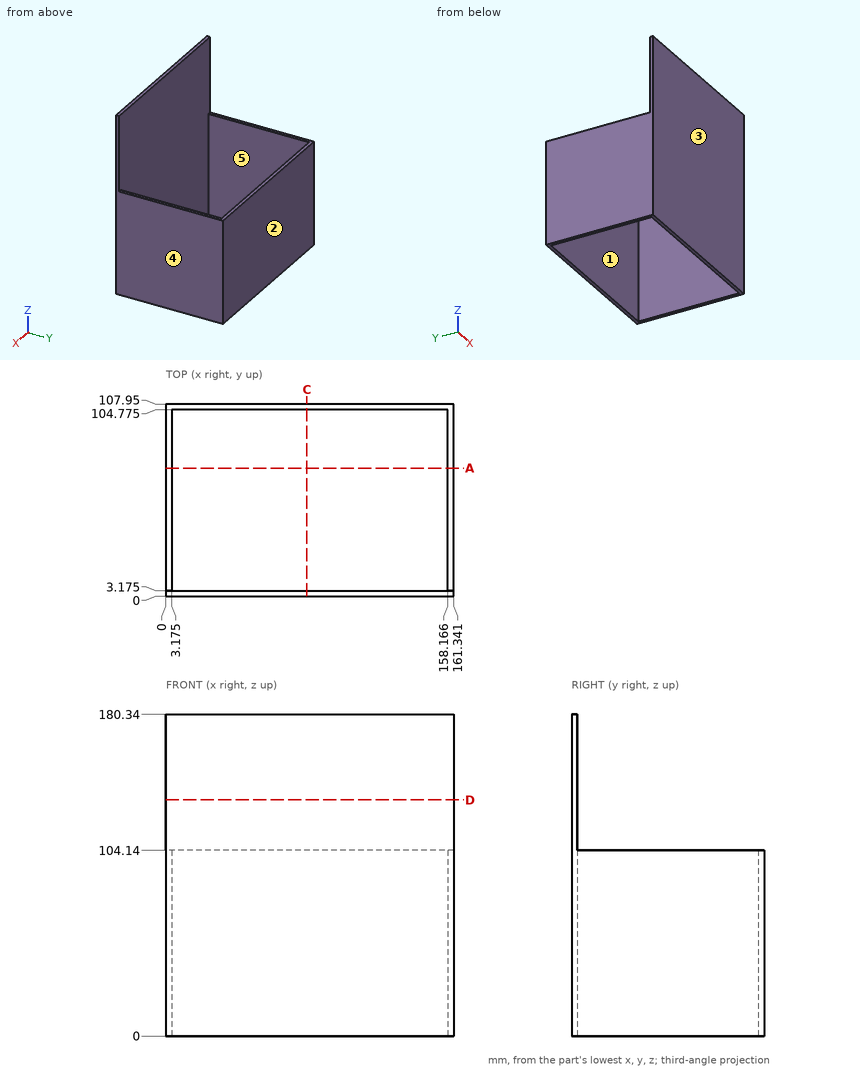
Geometry check sheet. Reference: drawing and pictorial views, mm from the part's lowest x, y, z. A direction names the side the tool comes from. Round coordinates to 2 decimals unless told otherwise and drop trailing zeros. Loops run counter-clockwise (first coordinate to the right, second up) from the corner with the lowest first, then second, coordinate; pieces in that order, holes last. Notation, with made-up numbers: (61, -17.5) - (117, -17.5) arc R19 cw to (117, 19.5) - close; hole circle Ø2 at (33.5, -24). An arc over 180 degrees is marked (long way). Use a Markdown table: item, result. Add a question column.
1. Release check for a two-part mould opening along X. For the marked faces 3, 4 and 5 record: released by +X, released by -X, zero draft, split by the parting line, or undercut.
2. Section check A-A, the plane y = 72. Record the boundary of the cut face in (x, z) (1 decimal), plus the area to 3 significant figures.
3. Gauge pin test, flat ends, axial feed: pin 1 (12 mm diameter, centred on y = 56, z = 44.5, fed in from -X); pin 2 (3 mm diameter, centred on x = 114.5, z = 147, fed in from +Y) (3 decimals). Record the tip position at first contact, or that the pin passes through.
4. Thickness scan on probe 1 along Y at (x, z) = (93.5, 21.5) (3 decimals); probe 2 along X at (y, z) = (96, 89) (1 decimal); probe 3 along Y at (x, z) = (36.5, 134) (3 decimals). Record the ranges inside material, lowest first. Write a range as [from, to].
5. Section check D-D, the plane z = 132.5. Record the boundary of the cut face in (x, y) (1 decimal), plus the area to 3 significant figures.
6. Section check C-C, the plane x = 79. Record the boundary of the cut face in (y, z) (3 decimals).
7. Access from +Z, -Z, +X, -X, +Y, -Y to the whole of each face (thin tool, end or side, straight path). Record for the marked faces 1 and 2.
Checks:
| question | item | result |
|---|---|---|
| 1 | face 3 | zero draft |
| 1 | face 4 | released by +X |
| 1 | face 5 | undercut |
| 2 | outline | (0, 0) - (3.2, 0) - (3.2, 104.1) - (0, 104.1) - close; (158.2, 0) - (161.3, 0) - (161.3, 104.1) - (158.2, 104.1) - close |
| 2 | area | 661 mm^2 |
| 3 | pin 1 | stops at x = 0 |
| 3 | pin 2 | stops at y = 3.175 |
| 4 | probe 1 | y = [0, 3.175], [104.775, 107.95] |
| 4 | probe 2 | x = [0, 3.2], [158.2, 161.3] |
| 4 | probe 3 | y = [0, 3.175] |
| 5 | outline | (0, 0) - (161.3, 0) - (161.3, 3.2) - (0, 3.2) - close |
| 5 | area | 512 mm^2 |
| 6 | outline | (0, 0) - (3.175, 0) - (3.175, 180.34) - (0, 180.34) - close; (104.775, 0) - (107.95, 0) - (107.95, 104.14) - (104.775, 104.14) - close |
| 7 | face 1 | +Z, -Z |
| 7 | face 2 | +Z, -Z, +X, -X, +Y |
